Here's the drawing with two shaded views (mm, measured from the low corner). I have some questions. Give positions to 0.01 mm unless a question says otherwise; leave off trailing zeros. Loops run counter-clockwise (first coordinate to the right, second up) from the corner with the lowest first, then second, coordinate; pieces in that order, holes last. Notation, with made-up numbers: M 5,57 L 20,57 A14 cw 20,75 Z; hole C -14,-7.5 d10. An arc over 180 degrees is marked long. Put each result on its own line as item: value. Start each with the question number.
1) Please list where these lines run through material, in increasing order: line 1 along Z through (x, y) = (6.35, 1.4); line 2 along X through (y, z) = (2.9, 32.5); line 3 along X through (y, z) = (0.4, 6). Write a range as from..to.
2) Imagine slicing it at C-C (z = 16). Write out the boundary of the cut face in (x, y) (3 decimals).
3) Imagine slicing it at A-A (x = 6.35). Write out the boundary of the cut face in (y, z) (1 decimal), then the cut area to 3 significant figures.
4) For P1, Ø1, axis at x = 4.5, y = 2, coming from the +Z side; P2, Ø1, axis at y = 2.5, z = 17, coming from the +X side; P3, Ø3, axis at x = 6.35, z = 32.258, coming from the -Y side; P4, Ø1.6, axis at y = 1.5, z = 47, coming from the -X side, each with a flat end and sliding along its axis, tell me the tip position at first contact or that it passes through.
5) Imagine slicing it at B-B (y = 1.5). State how many separate pieces and enclosed holes the cut face has, then the cut area to 3 significant figures.
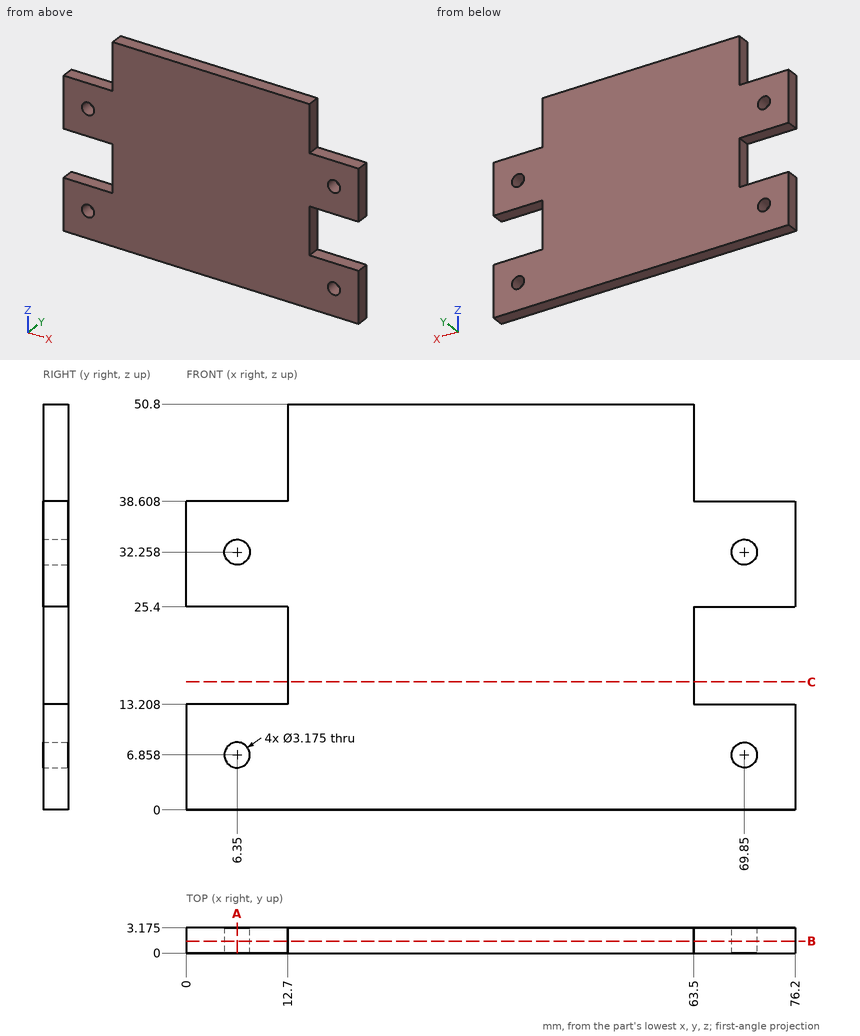
Recorded:
1. line 1: 0..5.27, 8.45..13.21, 25.4..30.67, 33.85..38.61
1. line 2: 0..4.78, 7.92..68.28, 71.42..76.2
1. line 3: 0..5.01, 7.69..68.51, 71.19..76.2
2. outline: M 12.7,0 L 63.5,0 L 63.5,3.175 L 12.7,3.175 Z
3. outline: M 0,0 L 3.2,0 L 3.2,5.3 L 0,5.3 Z; M 0,8.4 L 3.2,8.4 L 3.2,13.2 L 0,13.2 Z; M 0,25.4 L 3.2,25.4 L 3.2,30.7 L 0,30.7 Z; M 0,33.8 L 3.2,33.8 L 3.2,38.6 L 0,38.6 Z
3. area: 63.7 mm²
4. P1: z = 38.61
4. P2: x = 63.5
4. P3: through
4. P4: x = 12.7
5. separate pieces: 1
5. enclosed holes: 4
5. area: 3,220 mm²
